Could you check a few things on this drawing? It's one solid part, dimensions in mm from its lowest x, y, z. Give positions to 0.01 mm unless a question says otherwise; leave off trailing zeros. Order: outer loops, then holes, each group sorted by start corner. A loop starts at its lowest first (then second) coordinate and runs counter-clockwise, first axis right, second up.
Item 1: I want a section at B-B, the plane y = 0.4. Count the separate pieces of the cut face and the enclosed holes in it, then the cut area to 3 significant figures.
Item 2: I want a section at D-D, the plane z = 28. Write out the boundary of the cut face in (x, y).
Item 3: I want a section at C-C, the plane z = 14. Write out the boundary of the cut face in (x, y), then the cut area to 3 significant figures.
Item 4: I want a section at A-A, the plane x = 22. Write out the boundary of the cut face in (y, z).
Item 5: If I drill on line 1 along Z through (x, y) = (12, 0.9); line 2 along Z through (x, y) = (11.5, 0.9) (1 decimal); line 3 along X through (y, z) = (0.45, 17), over which ranges is the centre line in solid material (lowest first)?
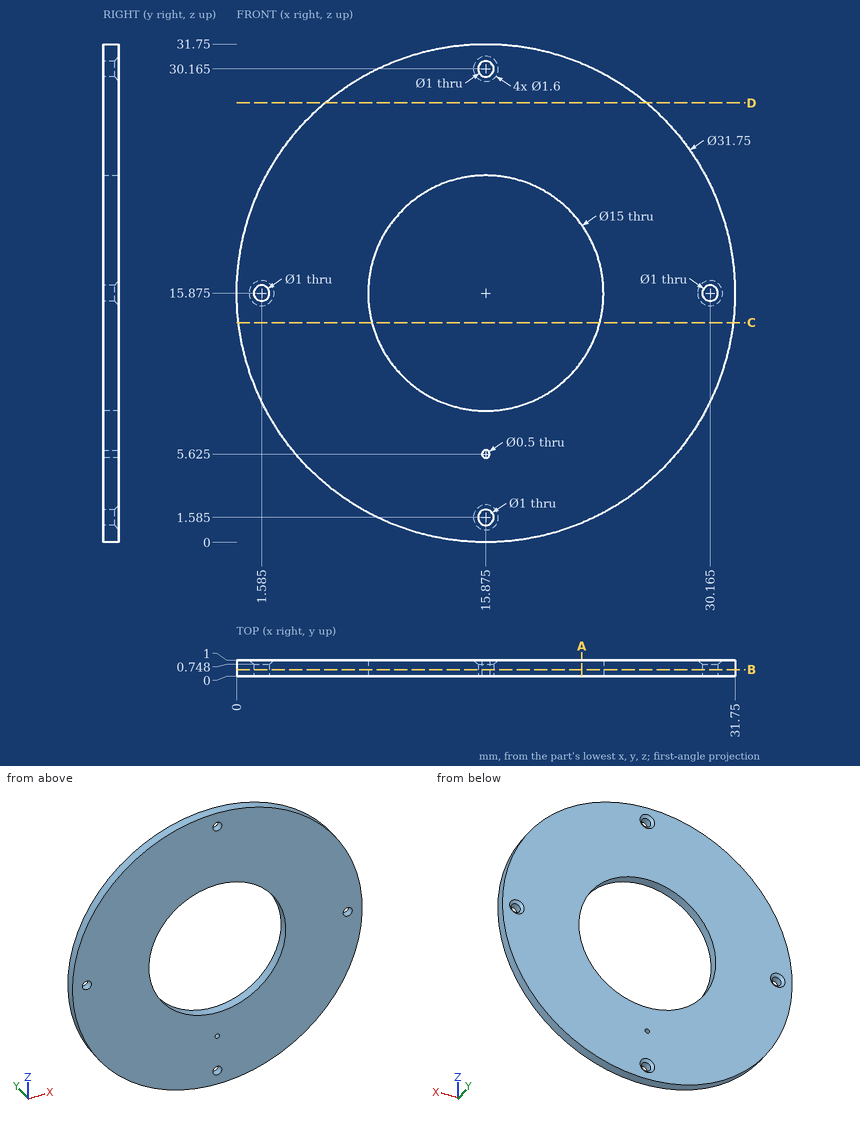
Results list:
1. separate pieces: 1
1. enclosed holes: 6
1. area: 612 mm2
2. outline: (5.63, 0) - (26.12, 0) - (26.12, 1) - (5.63, 1) - close
3. outline: (0.11, 0) - (8.61, 0) - (8.61, 1) - (0.11, 1) - close; (23.14, 0) - (31.64, 0) - (31.64, 1) - (23.14, 1) - close
3. area: 17.0 mm2
4. outline: (0, 1.23) - (1, 1.23) - (1, 11.55) - (0, 11.55) - close; (0, 20.2) - (1, 20.2) - (1, 30.52) - (0, 30.52) - close
5. line 1: z = 0.48 to 9.45, 22.3 to 31.27
5. line 2: z = 0.6 to 9.8, 22 to 31.1
5. line 3: x = 0.04 to 8.46, 23.29 to 31.71
